Input: part model. Units: mm. Frame: model coordinates. Give positions to 0.01 mm unless a question says otherwise; leave off trailing zeros. Loops run counter-clockwise (first coordinate to the right, second up) from the corner with the lowest first, then second, coordinate; pieces in that order, holes last. Notation, with made-up numbers: (-9.5, 44.5) - (38.5, 44.5) arc R21 ccw to (38.5, 49.5) - close; hole circle Ø10 at (-24, -27). An arc over 180 degrees is marked (long way). One line per item, written item: value.
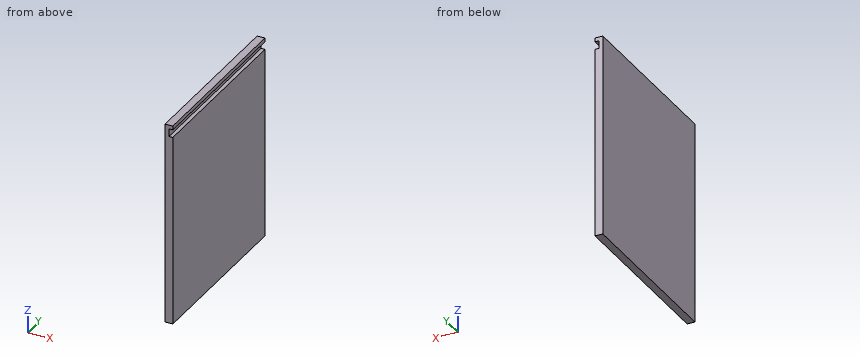
from build123d import *

# Parameters (mm, degrees)
F0_W     = 292.1
F0_H     = 304.8
F1_DEPTH = 12.7
F2_W     = 292.1
F2_H     = 25.4
F3_DEPTH = 12.7
F4_W     = 292.1
F4_H     = 12.7
F5_DEPTH = 6.35


with BuildPart() as f1:
    # F0 (on Right) → F1 (new body)
    with BuildSketch(Plane.YZ):
        with Locations((-146.05, 152.4)):
            Rectangle(F0_W, F0_H)
    extrude(amount=F1_DEPTH)

    # F2 (on Right) → F3 (join)
    with BuildSketch(Plane.YZ):
        with Locations((-146.05, -12.7)):
            Rectangle(F2_W, F2_H)
    extrude(amount=F3_DEPTH)

    # F4 (on face) → F5 (cut)
    with BuildSketch(Plane.YZ.offset(12.7)):
        with Locations((-146.05, 292.1)):
            Rectangle(F4_W, F4_H)
    extrude(amount=-F5_DEPTH, mode=Mode.SUBTRACT)


solid = f1.part
Item 1: Section B-B, the plane y = -258.5. Output: boundary loops of the cut face in (x, z), and give its area (3 significant figures).
Verdict:
outline: (0, -25.4) - (12.7, -25.4) - (12.7, 285.75) - (6.35, 285.75) - (6.35, 298.45) - (12.7, 298.45) - (12.7, 304.8) - (0, 304.8) - close
area: 4,110 mm^2
Item 2: Pin query (flat end, axial travel): P1, Ø10, axis at y = -112.5, z = 292, coming from the +X side. Return the tip coordinate at first contact, or that it passes through.
Verdict:
P1: stops at x = 6.35
Item 3: Material intervals for L1, parallel to Z at x = 11, y = -168.5; L2, parallel to X at y = -43, z = 291.5, sorted ascending.
Verdict:
L1: z = -25.4 to 285.75, 298.45 to 304.8
L2: x = 0 to 6.35
Item 4: Section A-A, the plane x = 8.5. Output: boundary loops of the cut face in (y, z), and give its area (3 significant figures).
Verdict:
outline: (-292.1, -25.4) - (0, -25.4) - (0, 285.75) - (-292.1, 285.75) - close; (-292.1, 298.45) - (0, 298.45) - (0, 304.8) - (-292.1, 304.8) - close
area: 92,700 mm^2
